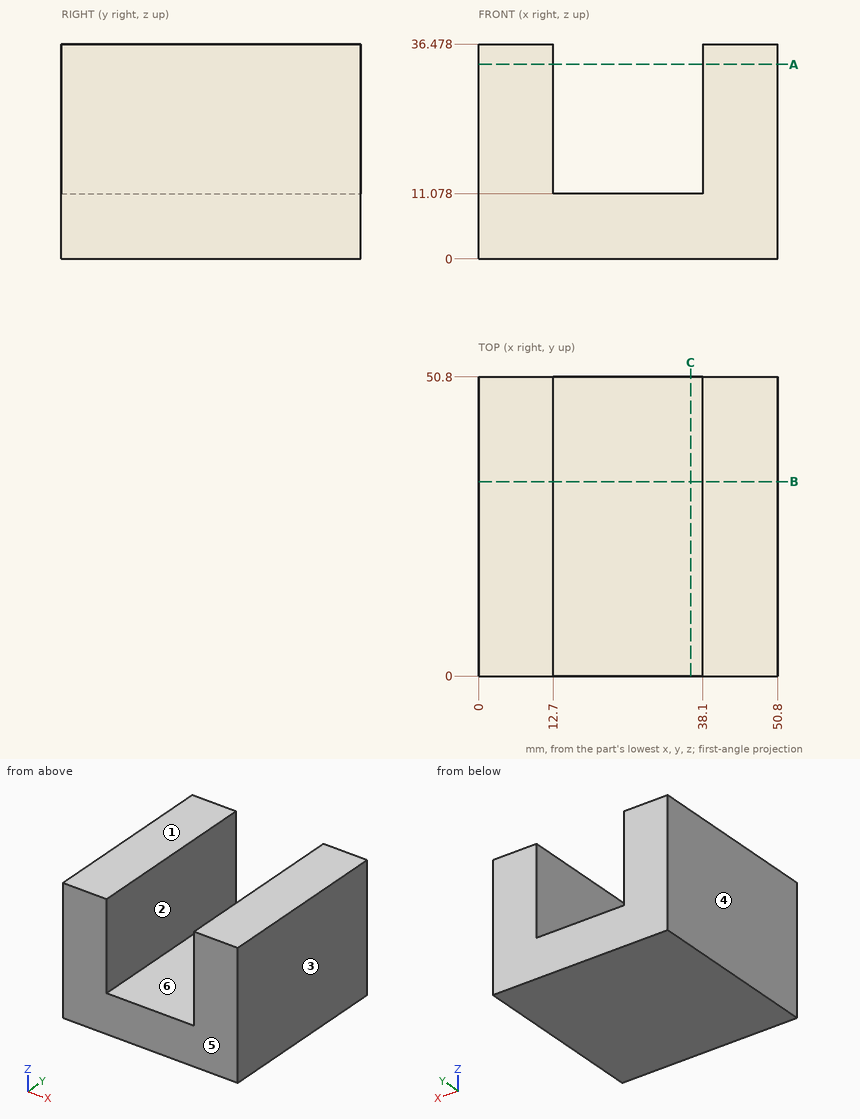
Here's the drawing with two shaded views (mm, measured from the low corner). I have some questions. A direction names the side the tool comes from. Round coordinates to 2 decimals unless told otherwise and drop trailing zeros. Loops run counter-clockwise (first coordinate to the right, second up) from the corner with the lowest first, then second, coordinate; pieces in that order, holes last. Notation, with made-up numbers: (30.25, -16.5) - (79.25, -16.5) arc R13 cw to (79.25, -8.5) - close; hole circle Ø1 at (11, 84). An arc over 180 degrees is marked (long way). Use CSV: the item, a comma, the result in double quotes. Start each with the question number.
1) For pin 1 Ø8 at (x, y) = (19, 17) entering from +Z, with a flat end and sliding along its axis, tell me the tip position at first contact or that it passes through.
2) For the marked faces 5 and 6, which set-ups out of +Z, -Z, +X, -X, +Y, -Y let a thin tool reach every point of the face, with its end or its side?
3) Please list where these lines run through material, in increasing order: probe 1 along X at (y, z) = (5.5, 35); probe 2 along Z at (x, y) = (31.5, 21). Write a range as [from, to].
4) We'd pull the mould along X, two halves only. Please class the marked faces 1, 2, 3 and 4: released by +X, released by -X, zero draft, split by the parting line, or undercut.
5) If we section it at A-A on z = 33: Write out the boundary of the cut face in (x, y), plus the area to 3 significant figures.
6) If we section it at C-C on x = 36: Write out the boundary of the cut face in (y, z).
7) If we section it at B-B on y = 33: Write out the boundary of the cut face in (x, z), plus the area to 3 significant figures.
Geometry results:
1,pin 1,"stops at z = 11.08"
2,face 5,"+Z, -Z, +X, -X, -Y"
2,face 6,"+Z, +Y, -Y"
3,probe 1,"x = [0, 12.7], [38.1, 50.8]"
3,probe 2,"z = [0, 11.08]"
4,face 1,"zero draft"
4,face 2,"undercut"
4,face 3,"released by +X"
4,face 4,"released by -X"
5,outline,"(0, 0) - (12.7, 0) - (12.7, 50.8) - (0, 50.8) - close; (38.1, 0) - (50.8, 0) - (50.8, 50.8) - (38.1, 50.8) - close"
5,area,"1,290 mm2"
6,outline,"(0, 0) - (50.8, 0) - (50.8, 11.08) - (0, 11.08) - close"
7,outline,"(0, 0) - (50.8, 0) - (50.8, 36.48) - (38.1, 36.48) - (38.1, 11.08) - (12.7, 11.08) - (12.7, 36.48) - (0, 36.48) - close"
7,area,"1,210 mm2"
